Model file for the job. Use its own axes, mm. A direction names the side the tool comes from. Round coordinates to 2 decimals unless told otherwise and drop trailing zeros. Loops run counter-clockwise (first coordinate to the right, second up) from the corner with the lowest first, then second, coordinate; pieces in that order, holes last. Notation, with made-up numbers: M 46.25,4 L 80.25,4 A27 ccw 80.25,32 Z; hole C -31,-2.75 d8. An arc over 180 degrees is marked long. Use a Markdown table: item, result. Add a question column.
Item 1: Saw through at A-A on z = 0. Write the cut outline in (x, y).
Item 2: Wall check: L1, parallel to Y at x = 175, z = 14.7; L2, parallel to Y at x = 172.7, z = 0; L3, parallel to Z at x = 171, y = -9. Give the ranges that are in metal, low to high. Write a range as from..to.
Item 3: Tool access for faces 4 (the cylindrical face through (171.82, -24.35, 15.92)), 5 (the cylindrical face through (172.235, -7.69, 24.418)), 6 (the flat face through (174, 24, 13)): list every direction of +Z, -Z, +X, -X, +Y, -Y with a clear straight run to the whole face (end or side of a thin tool).
Item 4: Pin check, flat tips, straight feed: P1, Ø3, axis at x = 175.5, y = 6, coming from the -Z side; P2, Ø4, axis at y = 25.46, z = 14.7, coming from the +X side; P3, Ø3, axis at x = 174, z = 19, coming from the -Y side. Stop position of each tip, or through.
Item 5: Two-plate mould, pull along Z, no slides. Class faces 1 (the cylindrical face through (175.331, 22.532, 15.35)), 2 (the flat face through (169.7, -26, 0)), 3 (the cylindrical face through (173.151, -1.513, -34.367)): +Z half, -Z half, draft (parallel to the pull), parting line (faces both ways), or undercut.
Item 6: Saw through at B-B on y = 0. Write the cut outline in (x, z).
Item 7: Saw through at D-D on z = 14.7. Write the cut outline in (x, y).
Item 8: Saw through at C-C on y = -10. Write the cut outline in (x, z), then the cut area to 3 significant figures.
```python
from build123d import *

# Parameters (mm, degrees)
AXIAL_HOLES_DEPTH      = 184.274684558
AXIAL_HOLES_DEPTH_BACK = 184.274684558
SKETCH2_R              = 1.65
CUT_EXTRUDE2_START     = 174
SKETCH3_R              = 3
CUT_EXTRUDE2_DEPTH     = 2.7


with BuildPart() as part:
    # Axial profile (mm) → Full revolution (revolve)
    with BuildSketch(Plane.XY, mode=Mode.PRIVATE) as full_revolution_sk:
        Polygon((169.7, 25.6), (174.7, 25.6), (174.7, 24), (176.7, 24), (176.7, 34.4), (169.7, 34.4), align=None)
    revolve(full_revolution_sk.sketch.rotate(Axis((-110, 0, 0), (1, 0, 0)), 90), axis=Axis((-110, 0, 0), (1, 0, 0)))

    # Sketch2 → Axial holes (cut, two sides: drawn at the far end of the back side and taken through both)
    with BuildSketch(Plane(origin=(0, 0, 0), x_dir=(0, 0, -1), z_dir=(1, 0, 0)).offset(-AXIAL_HOLES_DEPTH_BACK)):
        with Locations((29.4, 0)):
            Circle(SKETCH2_R)
        with Locations((-14.7, 25.461146871)):
            Circle(SKETCH2_R)
        with Locations((-14.7, -25.461146871)):
            Circle(SKETCH2_R)
    extrude(amount=AXIAL_HOLES_DEPTH + AXIAL_HOLES_DEPTH_BACK, mode=Mode.SUBTRACT)

    # Sketch3 → Cut-Extrude2 (cut)
    with BuildSketch(Plane(origin=(0, 0, 0), x_dir=(0, 0, -1), z_dir=(1, 0, 0)).offset(CUT_EXTRUDE2_START)):
        with Locations((29.4, 0)):
            Circle(SKETCH3_R)
        with Locations((-14.7, 25.461146871)):
            Circle(SKETCH3_R)
        with Locations((-14.7, -25.461146871)):
            Circle(SKETCH3_R)
    extrude(amount=CUT_EXTRUDE2_DEPTH, mode=Mode.SUBTRACT)


solid = part.part
```
Entries:
| question | item | result |
|---|---|---|
| 1 | outline | M 169.7,-34.4 L 176.7,-34.4 L 176.7,-24 L 174.7,-24 L 174.7,-25.6 L 169.7,-25.6 Z; M 169.7,25.6 L 174.7,25.6 L 174.7,24 L 176.7,24 L 176.7,34.4 L 169.7,34.4 Z |
| 2 | L1 | -31.1..-28.46, -22.46..-18.97, 18.97..22.46, 28.46..31.1 |
| 2 | L2 | -34.4..-25.6, 25.6..34.4 |
| 2 | L3 | -33.2..-23.97, 23.97..33.2 |
| 3 | face 4 | +X, -X |
| 3 | face 5 | -X |
| 3 | face 6 | +X |
| 4 | P1 | z = -34.1 |
| 4 | P2 | x = 174 |
| 4 | P3 | y = -29.62 |
| 5 | face 1 | undercut |
| 5 | face 2 | draft |
| 5 | face 3 | parting line |
| 6 | outline | M 169.7,-34.4 L 176.7,-34.4 L 176.7,-32.4 L 174,-32.4 L 174,-31.05 L 169.7,-31.05 Z; M 169.7,-27.75 L 174,-27.75 L 174,-26.4 L 176.7,-26.4 L 176.7,-24 L 174.7,-24 L 174.7,-25.6 L 169.7,-25.6 Z; M 169.7,25.6 L 174.7,25.6 L 174.7,24 L 176.7,24 L 176.7,34.4 L 169.7,34.4 Z |
| 7 | outline | M 169.7,-31.1 L 176.7,-31.1 L 176.7,-28.46 L 174,-28.46 L 174,-27.11 L 169.7,-27.11 Z; M 169.7,-23.81 L 174,-23.81 L 174,-22.46 L 176.7,-22.46 L 176.7,-18.97 L 174.7,-18.97 L 174.7,-20.96 L 169.7,-20.96 Z; M 169.7,20.96 L 174.7,20.96 L 174.7,18.97 L 176.7,18.97 L 176.7,22.46 L 174,22.46 L 174,23.81 L 169.7,23.81 Z; M 169.7,27.11 L 174,27.11 L 174,28.46 L 176.7,28.46 L 176.7,31.1 L 169.7,31.1 Z |
| 8 | outline | M 169.7,-32.91 L 176.7,-32.91 L 176.7,-21.82 L 174.7,-21.82 L 174.7,-23.57 L 169.7,-23.57 Z; M 169.7,23.57 L 174.7,23.57 L 174.7,21.82 L 176.7,21.82 L 176.7,32.91 L 169.7,32.91 Z |
| 8 | area | 138 mm2 |
